```python
from build123d import *

# Parameters (mm, degrees)
F0_R     = 18
F0_R_2   = 5
F1_DEPTH = 27
F0_R_3   = 3.95
F0_R_4   = 2.05
F2_DEPTH = 10
F3_DEPTH = 4


with BuildPart() as f1:
    # F0 (on Top) → F1 (new body)
    with BuildSketch(Plane.XY):
        with Locations((22, -22)):
            Circle(F0_R)
        with Locations((22, -22)):
            Circle(F0_R_2, mode=Mode.SUBTRACT)
    extrude(amount=-F1_DEPTH)

    # F0 (on Top) → F2 (join)
    with BuildSketch(Plane.XY):
        with BuildLine():
            Line((37.652476, 0), (6.347524, 0))
            ThreePointArc((6.347524, 0), (2.908117, -2.908117), (0, -6.347524))
            Line((0, -6.347524), (0, -37.652476))
            ThreePointArc((0, -37.652476), (2.908117, -41.091883), (6.347524, -44))
            Line((6.347524, -44), (37.652476, -44))
            ThreePointArc((37.652476, -44), (41.091883, -41.091883), (44, -37.652476))
            Line((44, -37.652476), (44, -6.347524))
            ThreePointArc((44, -6.347524), (41.091883, -2.908117), (37.652476, 0))
        make_face()
        with Locations((6.443651, -37.556349)):
            Circle(F0_R_3, mode=Mode.SUBTRACT)
        with Locations((37.556349, -37.556349)):
            Circle(F0_R_3, mode=Mode.SUBTRACT)
        with Locations((6.443651, -6.443651)):
            Circle(F0_R_3, mode=Mode.SUBTRACT)
        with Locations((22, -22)):
            Circle(F0_R, mode=Mode.SUBTRACT)
        with Locations((37.556349, -6.443651)):
            Circle(F0_R_3, mode=Mode.SUBTRACT)
        with Locations((6.443651, -6.443651)):
            Circle(F0_R_3)
        with Locations((6.443651, -6.443651)):
            Circle(F0_R_4, mode=Mode.SUBTRACT)
        with Locations((37.556349, -6.443651)):
            Circle(F0_R_3)
        with Locations((37.556349, -6.443651)):
            Circle(F0_R_4, mode=Mode.SUBTRACT)
        with Locations((37.556349, -37.556349)):
            Circle(F0_R_3)
        with Locations((37.556349, -37.556349)):
            Circle(F0_R_4, mode=Mode.SUBTRACT)
        with Locations((6.443651, -37.556349)):
            Circle(F0_R_3)
        with Locations((6.443651, -37.556349)):
            Circle(F0_R_4, mode=Mode.SUBTRACT)
    extrude(amount=-F2_DEPTH)

    # F0 (on Top) → F3 (cut)
    with BuildSketch(Plane.XY):
        with Locations((6.443651, -6.443651)):
            Circle(F0_R_3)
        with Locations((6.443651, -6.443651)):
            Circle(F0_R_4, mode=Mode.SUBTRACT)
        with Locations((37.556349, -6.443651)):
            Circle(F0_R_3)
        with Locations((37.556349, -6.443651)):
            Circle(F0_R_4, mode=Mode.SUBTRACT)
        with Locations((37.556349, -37.556349)):
            Circle(F0_R_3)
        with Locations((37.556349, -37.556349)):
            Circle(F0_R_4, mode=Mode.SUBTRACT)
        with Locations((6.443651, -37.556349)):
            Circle(F0_R_3)
        with Locations((6.443651, -37.556349)):
            Circle(F0_R_4, mode=Mode.SUBTRACT)
    extrude(amount=-F3_DEPTH, mode=Mode.SUBTRACT)


solid = f1.part
```
Model file for the job. Use its own axes, mm. A direction names the side the tool comes from. Round coordinates to 2 decimals unless told otherwise and drop trailing zeros. Write each loop counter-clockwise with the first axis right and the second up, starting at its lowest first coordinate (ties: lowest second). Pieces come first, ordered by that corner, then holes. Notation, with made-up numbers: M -37,74.5 L -6,74.5 A9 cw -6,79.5 Z; hole C 78.5,81 d9. An arc over 180 degrees is marked long. Put each result on its own line as item: value.
Item 1: Cut at C-C (z = -6.5). List the corners of the cut face in (x, y), and give its area (3 significant figures).
Responses:
outline: M 0,-37.65 A27 ccw 6.35,-44 L 37.65,-44 A27 ccw 44,-37.65 L 44,-6.35 A27 ccw 37.65,0 L 6.35,0 A27 ccw 0,-6.35 Z; hole C 6.44,-37.56 d4.1; hole C 6.44,-6.44 d4.1; hole C 22,-22 d10; hole C 37.56,-37.56 d4.1; hole C 37.56,-6.44 d4.1
area: 1,730 mm²
Item 2: Tool access for faces 4 (the cylindrical face through (8.567, -3.113, -1.972)), 5 (the flat face through (22, -44, -5)), 6 (the cylindrical face through (30.306, -37.969, -18.381)): list every direction of +Z, -Z, +X, -X, +Y, -Y with a clear straight run to the whole face (end or side of a thin tool).
Responses:
face 4: +Z
face 5: +Z, -Z, +X, -X, -Y
face 6: -Z
Item 3: Flat gauge pins, fed straight in: P1, Ø2, axis at x = 27.5, z = -10.5, coming from the -Y side; P2, Ø2, axis at y = -6.5, z = -12, coming from the +X side; P3, Ø3.5, axis at x = 6.44, y = -6.44, coming from the +Z side; P4, Ø1, axis at y = -20, z = -24, coming from the -X side. Where does each tip first touch, or does it go through?
Responses:
P1: y = -44
P2: x = 32.67
P3: through
P4: x = 4.06
Item 4: Probe L1, parallel to Y at x = 37, z = -6.25; L2, parallel to Z at x = 35, y = -9.5; L3, parallel to Y at x = 20, z = -11. List the from-to ranges inside material, lowest first. Write a range as from..to.
Responses:
L1: -44..-39.53, -35.58..-8.42, -4.47..0
L2: -10..0
L3: -39.89..-26.58, -17.42..-4.11
Item 5: Mould opens along X. For faces 1 (the flat face through (44, -22, -5)), 2 (the cylindrical face through (5.999, -8.445, -6.958)), 3 (the flat face through (22, 0, -5)) say: +X half, -X half, draft (parallel to the pull), parting line (faces both ways), or undercut.
Responses:
face 1: +X half
face 2: undercut
face 3: draft
Item 6: Cut at B-B (y = -22). List the corners of the cut face in (x, z).
Responses:
outline: M 0,-10 L 4,-10 L 4,-27 L 17,-27 L 17,0 L 0,0 Z; M 27,-27 L 40,-27 L 40,-10 L 44,-10 L 44,0 L 27,0 Z
Item 7: Cut at A-A (x = 22). List the corners of the cut face in (y, z), and give its area (3 significant figures).
Responses:
outline: M -44,-10 L -40,-10 L -40,-27 L -27,-27 L -27,0 L -44,0 Z; M -17,-27 L -4,-27 L -4,-10 L 0,-10 L 0,0 L -17,0 Z
area: 782 mm²
Item 8: Cut at D-D (y = -5). List the corners of the cut face in (x, z).
Responses:
outline: M 1.02,-10 L 4.99,-10 L 4.99,-4 L 2.77,-4 L 2.77,0 L 1.02,0 Z; M 7.9,-10 L 16.08,-10 L 16.08,-27 L 27.92,-27 L 27.92,-10 L 36.1,-10 L 36.1,-4 L 33.88,-4 L 33.88,0 L 10.12,0 L 10.12,-4 L 7.9,-4 Z; M 39.01,-10 L 42.98,-10 L 42.98,0 L 41.23,0 L 41.23,-4 L 39.01,-4 Z
